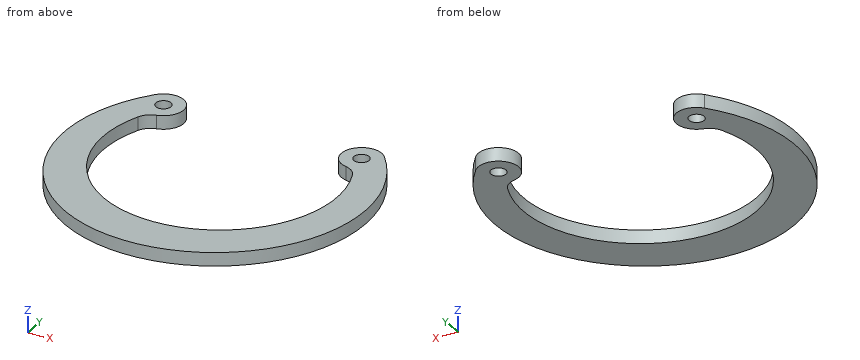
from build123d import *

# Parameters (mm, degrees)
SKETCH_1_R      = 0.85
EXTRUDE_1_DEPTH = 1.5


with BuildPart() as part:
    # Эскиз1 → Бобышка-Вытянуть1 (new body)
    with BuildSketch(Plane.XY):
        with BuildLine():
            ThreePointArc((-12.028004227, 5.932252459), (-11.46771854, 6.701660536), (-10.615237279, 7.124962483))
            ThreePointArc((-10.615237279, 7.124962483), (-9.185534057, 10.490032127), (-12.831244422, 10.766692462))
            ThreePointArc((-12.831244422, 10.766692462), (0, -16.75), (12.831244422, 10.766692462))
            ThreePointArc((12.831244422, 10.766692462), (9.185534057, 10.490032127), (10.615237279, 7.124962483))
            ThreePointArc((10.615237279, 7.124962483), (11.46771854, 6.701660536), (12.028004227, 5.932252459))
            ThreePointArc((12.028004227, 5.932252459), (0, -12), (-12.028004227, 5.932252459))
        make_face()
        with Locations((-11.107644425, 9.32042034)):
            Circle(SKETCH_1_R, mode=Mode.SUBTRACT)
        with Locations((11.107644425, 9.32042034)):
            Circle(SKETCH_1_R, mode=Mode.SUBTRACT)
    extrude(amount=-EXTRUDE_1_DEPTH)


solid = part.part
For this review, take the finished solid that the model builds, in its own axes (mm). Coordinates: 2 decimals unless noted, no trailing zeros. Order: outer loops, then holes, each group sorted by start corner. A loop starts at its lowest first (then second) coordinate and runs counter-clockwise, first axis right, second up. Notation, with made-up numbers: (65.25, 70.5) - (84.25, 70.5) arc R17 ccw to (84.25, 93.5) - close; hole circle Ø3 at (66.25, 32.25). An arc over 180 degrees is marked (long way). Answer as CSV lines item,"result". Start each with the question number.
1) Add section C-C (x = 0). State the section outline as (y, z) points.
2) To check wall thickness, follow line 1 along X through (y, z) = (9, -0.55); line 2 along X through (y, z) = (-10.75, -0.4); line 3 along X through (y, z) = (-9, -0.95). State the ranges of each line that lie inside material, in increasing order. Write a range as [from, to].
3) Add section B-B (z = -1.1). State the section outline as (x, y) points.
4) Add section A-A (y = -0.75). State the section outline as (x, z) points, then the cut area to 3 significant figures.
5) Add section D-D (y = -9). State the section outline as (x, z) points.
Result:
1,outline,"(-16.75, -1.5) - (-12, -1.5) - (-12, 0) - (-16.75, 0) - close"
2,line 1,"[-14.13, -11.89], [-10.32, -8.88], [8.88, 10.32], [11.89, 14.13]"
2,line 2,"[-12.85, -5.56], [5.56, 12.85]"
2,line 3,"[-14.13, -8.31], [8.31, 14.13]"
3,outline,"(-12.83, 10.77) arc R16.75 ccw (long way) to (12.83, 10.77) arc R2.25 ccw (long way) to (10.62, 7.12) arc R2 cw to (12.03, 5.93) arc R13 cw (long way) to (-12.03, 5.93) arc R2 cw to (-10.62, 7.12) arc R2.25 ccw (long way) to start; hole circle Ø1.7 at (-11.11, 9.32); hole circle Ø1.7 at (11.11, 9.32)"
4,outline,"(-16.73, -1.5) - (-12.88, -1.5) - (-12.88, 0) - (-16.73, 0) - close; (12.88, -1.5) - (16.73, -1.5) - (16.73, 0) - (12.88, 0) - close"
4,area,"11.6 mm^2"
5,outline,"(-14.13, -1.5) - (-8.31, -1.5) - (-8.31, 0) - (-14.13, 0) - close; (8.31, -1.5) - (14.13, -1.5) - (14.13, 0) - (8.31, 0) - close"
